Could you check a few things on this drawing? It's one solid part, dimensions in mm from its lowest x, y, z. Round coordinates to 2 decimals unless told otherwise and drop trailing zeros. Loops run counter-clockwise (first coordinate to the right, second up) from the corner with the lowest first, then second, coordinate; pieces in that order, holes last. Notation, with made-up numbers: (16.25, 75) -> (56.25, 75) arc R28 cw to (56.25, 111) -> close; hole circle Ø9 at (43, 5). An arc over 180 degrees is marked (long way). Use one line per item in the form item = value. Start each with the question number.
Item 1: If we section it at D-D (x = 43): Write out the boundary of the cut face in (y, z).
Item 2: Thinking about a two-plate mould opening in Y: for the marked faces 1, 2 and 3, which applies, released by +Y, released by -Y, zero draft, split by the parting line, or undercut?
Item 3: If we section it at A-A (x = 13): Write out the boundary of the cut face in (y, z), then the cut area to 3 significant figures.
Item 4: If I drill on L1, parallel to Y at x = 23, z = 5.75; L2, parallel to X at y = 9, z = 2.75; L3, parallel to Y at x = 43, z = 10, over which ranges is the centre line in solid material (lowest first)? Write a range as [from, to].
Item 5: If we section it at B-B (y = 10): Write out the boundary of the cut face in (x, z), then the cut area to 3 significant figures.
Item 6: If we section it at C-C (z = 9.75): Write out the boundary of the cut face in (x, y).
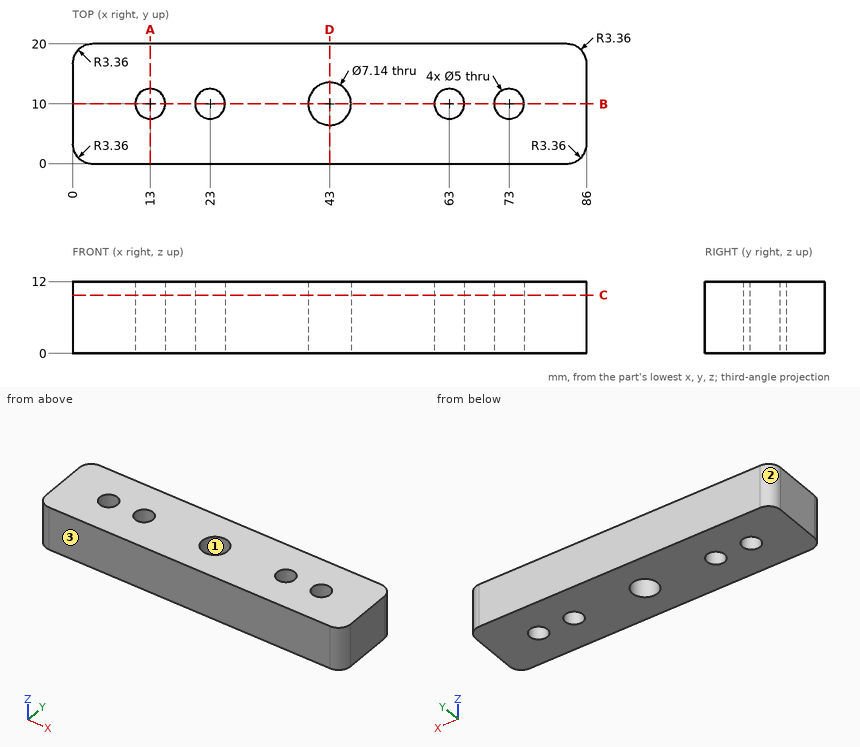
Values found:
q1.outline = (0, 0) -> (6.43, 0) -> (6.43, 12) -> (0, 12) -> close; (13.57, 0) -> (20, 0) -> (20, 12) -> (13.57, 12) -> close
q2.face_1 = undercut
q2.face_2 = released by +Y
q2.face_3 = released by -Y
q3.outline = (0, 0) -> (7.5, 0) -> (7.5, 12) -> (0, 12) -> close; (12.5, 0) -> (20, 0) -> (20, 12) -> (12.5, 12) -> close
q3.area = 180 mm2
q4.L1 = [0, 7.5], [12.5, 20]
q4.L2 = [0, 10.71], [15.29, 20.71], [25.29, 39.57], [46.43, 60.71], [65.29, 70.71], [75.29, 86]
q4.L3 = [0, 6.43], [13.57, 20]
q5.outline = (0, 0) -> (10.5, 0) -> (10.5, 12) -> (0, 12) -> close; (15.5, 0) -> (20.5, 0) -> (20.5, 12) -> (15.5, 12) -> close; (25.5, 0) -> (39.43, 0) -> (39.43, 12) -> (25.5, 12) -> close; (46.57, 0) -> (60.5, 0) -> (60.5, 12) -> (46.57, 12) -> close; (65.5, 0) -> (70.5, 0) -> (70.5, 12) -> (65.5, 12) -> close; (75.5, 0) -> (86, 0) -> (86, 12) -> (75.5, 12) -> close
q5.area = 706 mm2
q6.outline = (0, 3.36) arc R3.36 ccw to (3.36, 0) -> (82.64, 0) arc R3.36 ccw to (86, 3.36) -> (86, 16.64) arc R3.36 ccw to (82.64, 20) -> (3.36, 20) arc R3.36 ccw to (0, 16.64) -> close; hole circle Ø5 at (13, 10); hole circle Ø5 at (23, 10); hole circle Ø7.14 at (43, 10); hole circle Ø5 at (63, 10); hole circle Ø5 at (73, 10)
